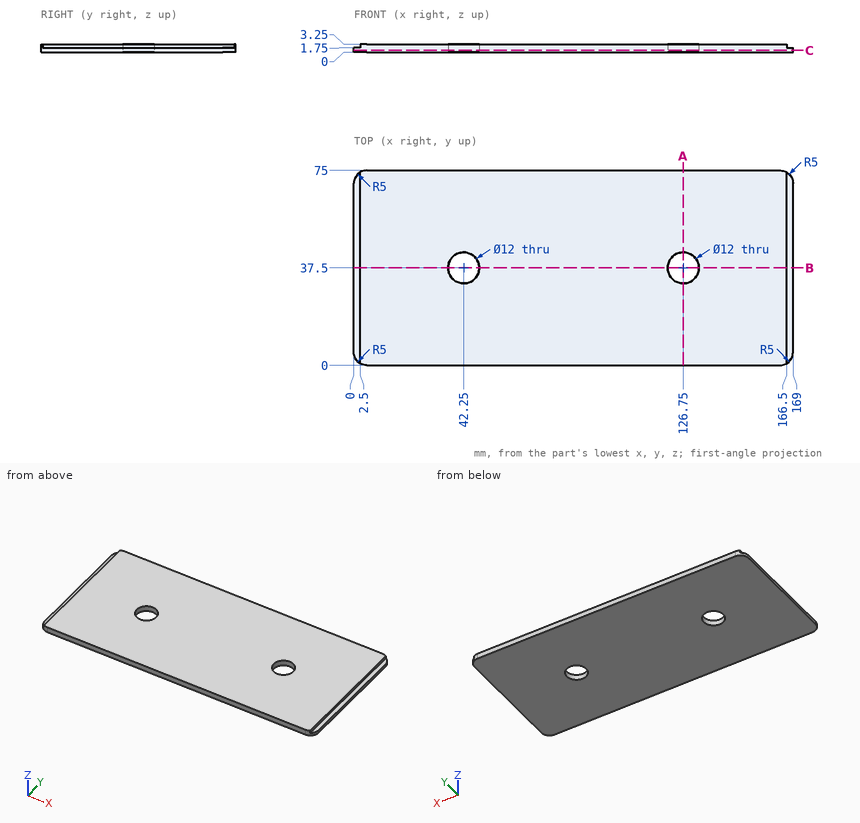
The drawing under review shows one solid part. Ordinate dimensions are in mm from its lowest x, y, z. Give positions to 0.01 mm unless a question says otherwise; leave off trailing zeros. Write each loop counter-clockwise with the first axis right and the second up, starting at its lowest first coordinate (ties: lowest second). Pieces come first, ordered by that corner, then holes.
1. Wall thickness on L1, parallel to X at y = 38, z = 2.4; L2, parallel to X at y = 37.5, z = 1.55; L3, parallel to Y at x = 42.25, z = 1.35: over which ranges is each line inside the solid? List them lowest first.
2. Add section B-B, the plane y = 37.5. Write out the cut boundary in (x, z).
3. Add section C-C, the plane z = 0.8. Write out the cut boundary in (x, y), plus the area to 3 significant figures.
4. Add section A-A, the plane x = 126.75. Write out the cut boundary in (y, z), plus the area to 3 significant figures.
5. For P1, Ø1.2, axis at x = 168, y = 48.5, coming from the +Z side, flat-tipped, find the tip position at first contact; note if it passes through.
Worked answers:
1. L1: x = 2.5 to 36.27, 48.23 to 120.77, 132.73 to 166.5
1. L2: x = 0 to 36.25, 48.25 to 120.75, 132.75 to 169
1. L3: y = 0 to 31.5, 43.5 to 75
2. outline: (0, 0) - (36.25, 0) - (36.25, 3.25) - (2.5, 3.25) - (2.5, 1.75) - (0, 1.75) - close; (48.25, 0) - (120.75, 0) - (120.75, 3.25) - (48.25, 3.25) - close; (132.75, 0) - (169, 0) - (169, 1.75) - (166.5, 1.75) - (166.5, 3.25) - (132.75, 3.25) - close
3. outline: (0, 5) arc R5 ccw to (5, 0) - (164, 0) arc R5 ccw to (169, 5) - (169, 70) arc R5 ccw to (164, 75) - (5, 75) arc R5 ccw to (0, 70) - close; hole circle Ø12 at (42.25, 37.5); hole circle Ø12 at (126.75, 37.5)
3. area: 12,400 mm2
4. outline: (0, 0) - (31.5, 0) - (31.5, 3.25) - (0, 3.25) - close; (43.5, 0) - (75, 0) - (75, 3.25) - (43.5, 3.25) - close
4. area: 205 mm2
5. P1: stops at z = 1.75
